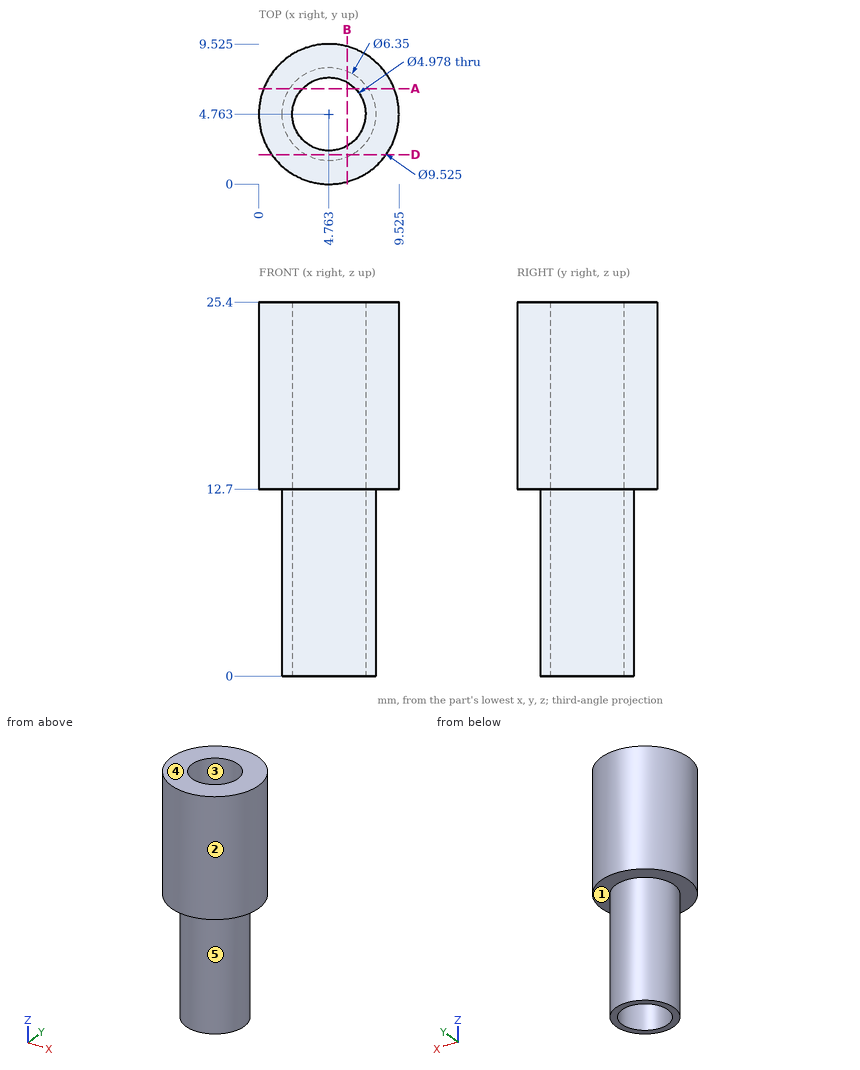
Answer from the drawing. Dimensions are ordinates in mm from the lowest x, y and z of the part. A direction names the side the tool comes from. Give positions to 0.01 mm unless a question says otherwise; leave off trailing zeros. Loops run counter-clockwise (first coordinate to the right, second up) from the corner with the lowest first, then second, coordinate; pieces in that order, holes last.
Item 1: The part is cut by section D-D (y = 2). Write down the section's boundary in (x, z).
Item 2: The mould has two halves that part along X. Classify the marked faces 1, 2 and 3: released by +X, released by -X, zero draft, split by the parting line, or undercut.
Item 3: The part is cut by section B-B (x = 6). Write down the section's boundary in (y, z).
Item 4: Each of these flat-tipped pins is pushed along its axis until it touches: pin 1 Ø5 at (x, z) = (7.5, 19.5) entering from -Y; pin 2 Ø1 at (x, z) = (3.5, 7) entering from +Y (1 decimal); pin 3 Ø2 at (x, z) = (4, 7) entering from +Y. Where does it stop, or does it pass through?
Item 5: The part is cut by section A-A (y = 6.5). Write down the section's boundary in (x, z) (1 decimal).
Item 6: For the marked faces 4 and 5, determine the directions among +Z, -Z, +X, -X, +Y, -Y from which every point of the face is accessible in a straight line to the end or side of a thin tool.
Item 7: Find the intervals of material crossed by line 1 along Y through (x, z) = (4.75, 4); line 2 along Z through (x, y) = (4, 9); line 3 along X through (y, z) = (4.75, 17.5) (1 decimal), in increasing order.
Taken from the geometry:
1. outline: (0.88, 12.7) - (3.2, 12.7) - (3.2, 0) - (6.33, 0) - (6.33, 12.7) - (8.64, 12.7) - (8.64, 25.4) - (0.88, 25.4) - close
2. face 1: zero draft
2. face 2: split by the parting line
2. face 3: undercut
3. outline: (0.16, 12.7) - (1.84, 12.7) - (1.84, 0) - (2.6, 0) - (2.6, 25.4) - (0.16, 25.4) - close; (6.92, 0) - (7.69, 0) - (7.69, 12.7) - (9.36, 12.7) - (9.36, 25.4) - (6.92, 25.4) - close
4. pin 1: stops at y = 0.01
4. pin 2: stops at y = 7.8
4. pin 3: stops at y = 7.94
5. outline: (0.3, 12.7) - (2.1, 12.7) - (2.1, 0) - (3, 0) - (3, 25.4) - (0.3, 25.4) - close; (6.5, 0) - (7.4, 0) - (7.4, 12.7) - (9.2, 12.7) - (9.2, 25.4) - (6.5, 25.4) - close
6. face 4: +Z, +X, -X, +Y, -Y
6. face 5: -Z
7. line 1: y = 1.59 to 2.27, 7.25 to 7.94
7. line 2: z = 12.7 to 25.4
7. line 3: x = 0 to 2.3, 7.3 to 9.5
